Can you work these out from the drawing? Everything is in mm from the part's minimum corner. Round coordinates to 2 decimals unless told otherwise and drop trailing zeros. Order: outer loops, then holes, each group sorted by start corner. A loop starts at its lowest first (then second) coordinate and runs counter-clockwise, first axis right, second up. Notation, with made-up numbers: M 3,-26 L 41,-26 A17 ccw 41,0 Z; hole C -2.75,26.25 d6. An arc over 180 degrees is marked long. Write each question's results on one line, items separated by ' | '. Start each with the question number.
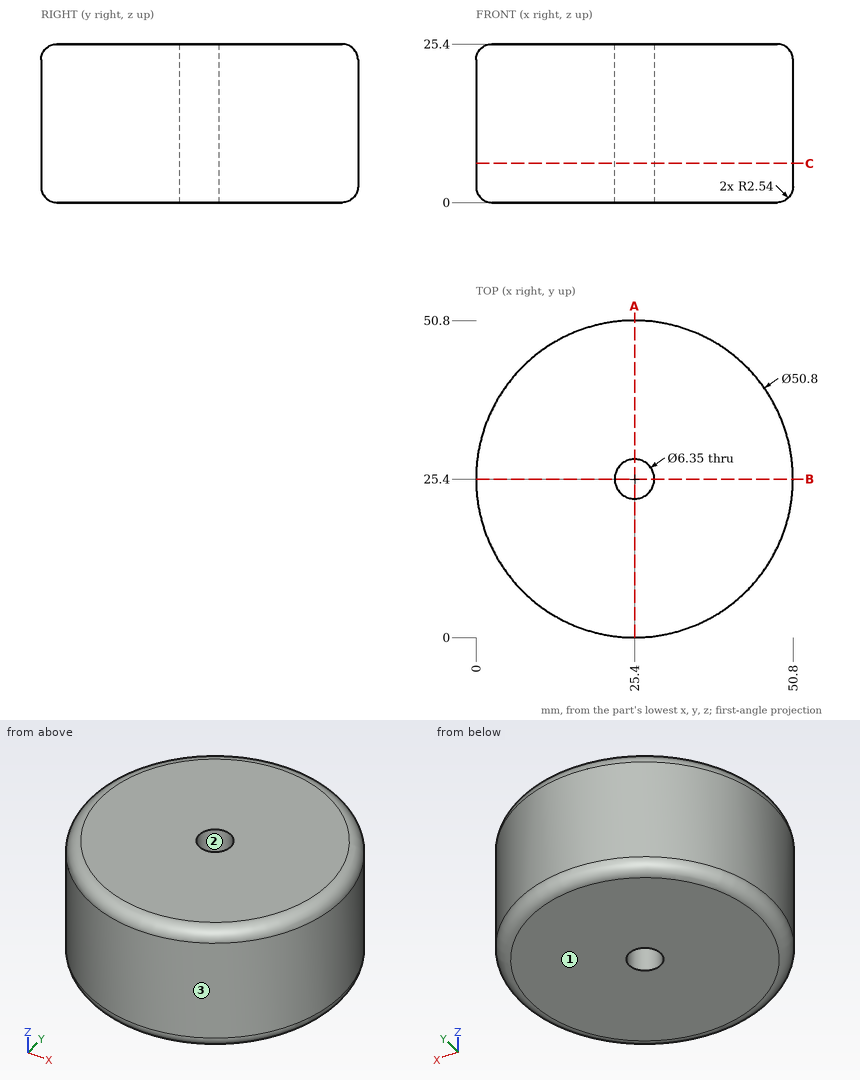
(1) I want a section at A-A on x = 25.4. Write out the boundary of the cut face in (y, z) (3 decimals), and give its area (3 significant figures).
(2) I'm going to push flat-ended pins straight in: pin 1 Ø6 at (y, z) = (5.5, 15.5) entering from +X; pin 2 Ø3 at (x, z) = (11.5, 19) entering from +Y; pin 3 Ø2 at (x, z) = (7, 5) entering from +Y. Where does each tip first touch, or does it pass through?
(3) Please list where these lines run through material, in increasing order: line 1 (Y direction, x = 24.5, z = 19.25); line 2 (Y direction, x = 25.4, z = 14) (3 decimals); line 3 (Y direction, x = 47.5, z = 11).
(4) If we mould it in two halves opening along Y, with no side actions, what happens to the marked faces 1, 2 and 3? For each: pulls with the +Y half, pulls with the -Y half, needs draft (parallel to the pull), parting line crosses it, or undercut.
(5) I want a section at C-C on z = 6.25. Write out the boundary of the cut face in (x, y) (3 decimals).
Solutions:
1) outline: M 0,2.54 A2.54 ccw 2.54,0 L 22.225,0 L 22.225,25.4 L 2.54,25.4 A2.54 ccw 0,22.86 Z; M 28.575,0 L 48.26,0 A2.54 ccw 50.8,2.54 L 50.8,22.86 A2.54 ccw 48.26,25.4 L 28.575,25.4 Z | area: 1,120 mm^2
2) pin 1: x = 44.36 | pin 2: y = 47.57 | pin 3: y = 43.9
3) line 1: 0.02 to 22.36, 28.44 to 50.78 | line 2: 0 to 22.225, 28.575 to 50.8 | line 3: 12.88 to 37.92
4) face 1: needs draft | face 2: undercut | face 3: parting line crosses it
5) outline: C 25.4,25.4 d50.8; hole C 25.4,25.4 d6.35
